For this review, take the finished solid that the model builds, in its own axes (mm). A direction names the side the tool comes from. Give positions to 0.01 mm unless a question says otherwise; leave off trailing zeros. Order: outer loops, then holes, each group sorted by start corner. A loop starts at its lowest first (then second) coordinate and runs counter-clockwise, first axis right, second up. Notation, with made-up numbers: (89, 60.25) - (142, 60.25) arc R17 ccw to (142, 86.25) - close; hole circle Ø2 at (85.5, 83.5). An arc over 180 degrees is marked (long way). Put each result on its own line as item: value. Start each with the question number.
```python
from build123d import *

# Parameters (mm, degrees)
SKETCH1_W           = 10
SKETCH1_H           = 2.5
BOSS_EXTRUDE1_DEPTH = 2.5


with BuildPart() as part:
    # Sketch1 → Boss-Extrude1 (new body)
    with BuildSketch(Plane.XY):
        Polygon((-24.5, -25), (-14.5, -25), (-14.5, -30), (-4.5, -30), (-4.5, -25), (4.5, -25), (4.5, -30), (14.5, -30), (14.5, -25), (24.5, -25), (24.5, 27.303543512), (14.5, 23.26200402), (14.5, 25.958460508), (4.5, 21.916921016), (4.5, 19.220464528), (-4.5, 15.583078984), (-4.5, 18.279535472), (-14.5, 14.23799598), (-14.5, 11.541539492), (-24.5, 7.5), align=None)
        with Locations((-9.5, 6.25)):
            Rectangle(SKETCH1_W, SKETCH1_H, mode=Mode.SUBTRACT)
        with Locations((9.5, 6.25)):
            Rectangle(SKETCH1_W, SKETCH1_H, mode=Mode.SUBTRACT)
        with BuildLine():
            Line((21, 21.017263456), (21, 11.5))
            ThreePointArc((21, 11.5), (20.707106781, 10.792893219), (20, 10.5))
            Line((20, 10.5), (-3.54860932, 10.5))
            ThreePointArc((-3.54860932, 10.5), (-4.530226027, 11.309137116), (-3.923317712, 12.427142719))
            Line((-3.923317712, 12.427142719), (19.625291609, 21.944406175))
            ThreePointArc((19.625291609, 21.944406175), (20.559147391, 21.846331725), (21, 21.017263456))
        make_face(mode=Mode.SUBTRACT)
    extrude(amount=BOSS_EXTRUDE1_DEPTH)


solid = part.part
```
1. Add section B-B, the plane x = 2. Give the boundary of the cut face in (y, z), then the cut area to 3 significant figures.
2. The part is to be moulded in two halves that separate along Y. For faces 4 (the face through (20.548, 21.854, 1.232)), 5 (the face through (0.063, 17.427, 1.232)), 6 (the face through (-14.5, -27, 1)), say which applies: released by +Y, released by -Y, zero draft, split by the parting line, or undercut.
3. Add section A-A, the plane z = 1.05. Count the separate pieces of the cut face and the enclosed holes in it, then the cut area to 3 significant figures.
4. Tool access review of faces 1 (the face through (-10, 5, 1)), 2 (the face through (19.57, 25.31, 1.23)), 3 (the face through (4.5, -27, 1)): name each direction out of +Z, -Z, +X, -X, +Y, -Y from which nothing blocks a thin tool from reaching the whole face with its end or side.
5. Wall thickness on line 1 (X direction, y = 17.5, z = 1.05); line 2 (X direction, y = 16.5, z = 1.6); line 3 (Y direction, x = 5.5, z = 1.9): over which ranges is each line inside the solid? List them lowest first. Write a range as from..to.
6. Add section C-C, the plane x = -19. Give the boundary of the cut face in (y, z).
7. Clearance check with flat-ended pins moving along their axes: pin 1 (1 mm diameter, centred on y = 11.5, z = 2, fed in from -X); pin 2 (0.8 mm diameter, centred on y = 12.5, z = 1, fed in from -X); pin 3 (0.8 mm diameter, centred on x = 2, z = 1.5, fed in from -Y); pin 4 (10 mm diameter, centred on x = 10, y = 14.5, fed in from +Z). State where each tip first meets the part, or that it passes through.
Found:
1. outline: (-25, 0) - (10.5, 0) - (10.5, 2.5) - (-25, 2.5) - close; (14.82, 0) - (18.21, 0) - (18.21, 2.5) - (14.82, 2.5) - close
1. area: 97.2 mm^2
2. face 4: undercut
2. face 5: released by +Y
2. face 6: zero draft
3. separate pieces: 1
3. enclosed holes: 3
3. area: 2,010 mm^2
4. face 1: +Z, -Z
4. face 2: +Z, -Z, +Y
4. face 3: +Z, -Z, -Y
5. line 1: x = -6.43..-4.5, 0.24..8.63, 21..24.5
5. line 2: x = -8.9..-4.5, -2.23..6.15, 21..24.5
5. line 3: y = -30..5, 7.5..10.5, 16.24..22.32
6. outline: (-25, 0) - (9.72, 0) - (9.72, 2.5) - (-25, 2.5) - close
7. pin 1: stops at x = -15.84
7. pin 2: stops at x = -14.5
7. pin 3: stops at y = -25
7. pin 4: stops at z = 2.5
